CAD build for the part. Positions are in the model's coordinates, mm. A direction names the side the tool comes from. Coordinates: 2 decimals unless noted, no trailing zeros. Order: outer loops, then holes, each group sorted by start corner. A loop starts at its lowest first (then second) coordinate and runs counter-clockwise, first axis right, second up. Notation, with made-up numbers: M 49.5,-37.5 L 59.5,-37.5 A10 cw 59.5,-29.5 Z; hole C 9.5,35 d2. An arc over 180 degrees is marked long. One line per item, written item: value.
Autodesk Inventor part; units mm, degrees
ref_plane "YZ Plane" through (0, 0, 0) normal (1, 0, 0) x (0, 1, 0)
ref_plane "XZ Plane" through (0, 0, 0) normal (0, 1, 0) x (-1, 0, 0)
ref_plane "XY Plane" through (0, 0, 0) normal (0, 0, 1) x (1, 0, 0)
sketch "Sketch2" plane through (0, 0, 0) normal (0, 0, 1) x (1, 0, 0)
  line L0 (-7, 4.75) -> (12.8, 4.75)
  line L1 (12.8, 4.75) -> (12.8, -4.75)
  line L2 (12.8, -4.75) -> (-7, -4.75)
  line L3 (-7, -4.75) -> (-7, 4.75)
  line L4 (-3.9, 4.75) -> (0.1, 4.75)
  line L5 (0.1, 4.75) -> (0.1, 5.15)
  line L6 (0.1, 5.15) -> (-3.9, 5.15)
  line L7 (-3.9, 5.15) -> (-3.9, 4.75)
  line L8 (5.6, 4.75) -> (9.6, 4.75)
  line L9 (9.6, 4.75) -> (9.6, 5.15)
  line L10 (9.6, 5.15) -> (5.6, 5.15)
  line L11 (5.6, 5.15) -> (5.6, 4.75)
  line L12 (-7, -4.75) -> (3, -4.75)
  line L13 (3, -4.75) -> (3, -5.45)
  line L14 (3, -5.45) -> (-7, -5.45)
  line L15 (-7, -5.45) -> (-7, -4.75)
  circle A0 centre (-1.9, 2.25) radius 1.15
  circle A1 centre (7.6, 2.25) radius 1.15
  point P0 (0, 0)
  dimension "d2" = 19.8
  dimension "d3" = 9.5
  dimension "d4" = 7
  dimension "d5" = 4.75
  dimension "d6" = 0.4
  dimension "d8" = 0.4
  dimension "d10" = 4
  dimension "d11" = 4
  dimension "d13" = 10
  dimension "d14" = 5.1
  dimension "d15" = 9.5
  dimension "d16" = 2
  dimension "d17" = 2
  dimension "d18" = 3.2
  dimension "d21" = 2.3
  dimension "d22" = 2.3
  dimension "d80" = 7.2
  dimension "d81" = 2.5
  dimension "d82" = 2.5
  dimension "d83" = 10.2
extrude "Extrusion1" add sketch "Sketch2" along normal mid plane 6
chamfer "Chamfer1" distance 0.4 angle 45 4 edges at (-3.9, 5.15, 0) (0.1, 5.15, 0) (5.6, 5.15, 0) (9.6, 5.15, 0)
chamfer "Chamfer3" distance 0.7 angle 45 1 edges at (3, -5.45, 0)
sketch "Sketch3" plane through (0, 0, 3) normal (0, 0, 1) x (1, 0, 0)
  line L0 (9.2, 5.15) -> (9.6, 4.75)
  line L1 (9.6, 5.15) -> (5.6, 5.15)
  line L2 (5.6, 4.75) -> (6, 5.15)
  line L3 (-0.3, 5.15) -> (0.1, 4.75)
  line L4 (0.1, 5.15) -> (-3.9, 5.15)
  line L5 (-3.9, 4.75) -> (-3.5, 5.15)
  circle A0 centre (7.6, 2.25) radius 1.15
  circle A1 centre (-1.9, 2.25) radius 1.15
  circle A2 centre (-1.9, 2.25) radius 2
  circle A3 centre (7.6, 2.25) radius 2
  line L6 (-3.9, 2.25) -> (-3.9, 4.75)
  line L7 (0.1, 2.25) -> (0.1, 4.75)
  line L8 (5.6, 2.25) -> (5.6, 4.75)
  line L9 (9.6, 2.25) -> (9.6, 4.75)
  point P0 (0, 0)
  dimension "d28" = 4
  dimension "d29" = 4
  dimension "d30" = 4
extrude "Extrusion2" add sketch "Sketch3" along normal blind 0.2
mirror "Mirror1" about plane through (0, 0, 0) normal (0, 0, 1) of "Extrusion2"
sketch "Sketch4" plane through (-7, -5.45, -3) normal (0, -1, 0) x (1, 0, 0)
  line L0 (6, 5) -> (8, 5)
  line L1 (8, 5) -> (8, 1)
  line L2 (8, 1) -> (6, 1)
  line L3 (6, 1) -> (6, 5)
  point P0 (7, 3)
  dimension "d33" = 2
  dimension "d34" = 4
  dimension "d35" = 1
  dimension "d36" = 2
extrude "Extrusion3" cut sketch "Sketch4" against normal blind 4
sketch "Sketch5" plane through (-7, 4.75, 3) normal (0, 1, 0) x (1, 0, 0)
  line L0 (7.1, 6) -> (12.6, 6)
  line L1 (12.6, 0) -> (7.1, 0)
  line L2 (19.6, 0) -> (16.4, 0)
  line L3 (16.4, 6) -> (19.6, 6)
  line L4 (1.3, 4.7) -> (1.8, 4.7)
  line L5 (1.8, 4.7) -> (1.8, 1.3)
  line L6 (1.8, 1.3) -> (1.3, 1.3)
  line L7 (1.3, 1.3) -> (1.3, 4.7)
  line L8 (10.1, 4.7) -> (10.6, 4.7)
  line L9 (10.6, 4.7) -> (10.6, 1.3)
  line L10 (10.6, 1.3) -> (10.1, 1.3)
  line L11 (10.1, 1.3) -> (10.1, 4.7)
  line L12 (-0.2, 3) -> (19.6, 3) construction
  line L13 (17.4, 4.7) -> (17.9, 4.7)
  line L14 (17.9, 4.7) -> (17.9, 1.3)
  line L15 (17.9, 1.3) -> (17.4, 1.3)
  line L16 (17.4, 1.3) -> (17.4, 4.7)
  line L17 (0, 0) -> (0, 6)
  line L18 (0, 6) -> (3.1, 6)
  line L19 (0, 0) -> (0, 6)
  line L20 (19.8, 0) -> (16.6, 0)
  line L21 (19.8, 6) -> (19.8, 0)
  line L22 (0, 6) -> (3.1, 6)
  line L23 (3.1, 0) -> (3.1, 6)
  line L24 (3.1, 0) -> (0, 0)
  line L25 (12.6, 0) -> (12.6, 6)
  line L26 (7.1, 6) -> (12.6, 6)
  line L27 (7.1, 6) -> (7.1, 0)
  line L28 (12.6, 0) -> (7.1, 0)
  line L29 (16.4, 6) -> (16.4, 0)
  line L30 (3.1, 0) -> (3.1, 6)
  line L31 (3.1, 0) -> (0, 0)
  line L32 (12.6, 0) -> (12.6, 6)
  line L33 (7.1, 6) -> (7.1, 0)
  line L34 (16.6, 6) -> (16.6, 0)
  line L35 (16.6, 6) -> (19.8, 6)
  line L36 (3.1, 0) -> (0.4, 0)
  line L37 (1.55, 4.7) -> (1.55, 1.3) construction
  line L38 (10.35, 4.7) -> (10.35, 1.3) construction
  line L39 (17.65, 4.7) -> (17.65, 1.3) construction
  point P0 (7, 3)
  dimension "d39" = 3.4
  dimension "d40" = 3.4
  dimension "d41" = 0.5
  dimension "d42" = 0.5
  dimension "d43" = 1.7
  dimension "d44" = 1.7
  dimension "d46" = 9.3
  dimension "d47" = 3.4
  dimension "d48" = 0.5
  dimension "d49" = 1.7
  dimension "d50" = 16.6
  dimension "d87" = 8.8
  dimension "d88" = 7.3
  dimension "d89" = 3.1
  dimension "d90" = 1.55
  dimension "d91" = 6
  dimension "d92" = 3
extrude "Extrusion4" add sketch "Sketch5" along normal blind 4 contours L4 L5 L6 L7 | L8 L9 L10 L11 | L13 L14 L15 L16
chamfer "Chamfer2" distance 0.5 angle 45 6 edges at (-5.45, 8.75, 1.7) (-5.45, 8.75, -1.7) (3.35, 8.75, -1.7) (3.35, 8.75, 1.7) (10.65, 8.75, -1.7) (10.65, 8.75, 1.7)
sketch "Sketch6" plane through (-5.7, 4.75, -1.7) normal (-1, 0, 0) x (0, 0, 1)
  line L0 (0, 0) -> (0, 3.5)
  line L1 (3.4, 0) -> (3.4, 3.5)
  line L2 (0.5, 4) -> (2.9, 4)
  point P0 (1.7, -4.75)
  point P1 (1.7, 2.5)
  dimension "d56" = 3.4
  dimension "d57" = 1.7
  dimension "d58" = 1.5
hole "Hole1" at (-5.7, 7.25, 0) direction (1, 0, 0) diameter 1.6 end through all
sketch "Sketch7" plane through (0, 0, 3) normal (0, 0, 1) x (1, 0, 0)
  line L0 (-7, 4.75) -> (-7, -5.45)
  line L1 (-7, -5.45) -> (3, -5.45)
  line L2 (-4, -5.45) -> (-4, -2.45) construction
  line L3 (-5.5, -5.45) -> (-5.5, -2.45)
  line L4 (-2.5, -2.45) -> (-2.5, -5.45)
  arc A0 (-5.5, -5.45) -> (-2.5, -5.45) centre (-4, -5.45) ccw
  arc A1 (-2.5, -2.45) -> (-5.5, -2.45) centre (-4, -2.45) ccw
  point P0 (2.6, -5.45)
  point P1 (0, 0)
  point P2 (-4, -3.95)
  dimension "d66" = 3
  dimension "d68" = 3
  dimension "d69" = 3
extrude "Extrusion5" cut sketch "Sketch7" against normal blind 0.5
sketch "Sketch8" plane through (0, 0, 2.5) normal (0, 0, 1) x (1, 0, 0)
  arc A0 (-2.5, -2.45) -> (-5.5, -2.45) centre (-4, -2.45) ccw
  circle A1 centre (-4, -2.45) radius 0.4
  point P0 (0, 0)
  dimension "d72" = 0.8
extrude "Extrusion6" add sketch "Sketch8" along normal up to surface (0.5 mm away)
mirror "Mirror2" about plane through (0, 0, 0) normal (0, 0, 1) of "Extrusion5", "Extrusion6"
sketch "Sketch9" plane through (0, 0, -3) normal (0, 0, -1) x (-1, 0, 0)
  arc A0 (5.5, -2.45) -> (2.5, -2.45) centre (4, -2.45) ccw
  line L0 (5.5, -2.45) -> (5.5, -5.45)
  line L1 (5.5, -5.45) -> (7, -5.45)
  line L2 (6.0521, -5.45) -> (5.4772, -2.1895)
  line L3 (6.0521, -5.45) -> (5.5, -5.45)
  point P0 (0, 0)
  dimension "d75" = 10
extrude "Extrusion7" cut sketch "Sketch9" against normal up to surface (0.5 mm away)
mirror "Mirror3" about plane through (0, 0, 0) normal (0, 0, 1) of "Extrusion7"
fillet "Fillet1" radius 0.5 2 edges at (12.8, -4.75, 0) (-7, -5.45, 0)
equation "\"d8\" = d6"
equation "\"d11\" = d10"
equation "\"d22\" = d21"
equation "\"d29\" = d28"
equation "\"d30\" = d29"
equation "\"d40\" = d39"
equation "\"d42\" = d41"
equation "\"d43\" = 0.5 * d39"
equation "\"d44\" = 0.5 * d40"
equation "\"d47\" = d39"
equation "\"d48\" = d41"
equation "\"d49\" = 0.5 * d47"
equation "\"d90\" = 0.5 * d89"
equation "\"d92\" = 0.5 * d91"
properties part number "KW-5A-125250V_body#" material "PC_ABS Plastic"
Q1. Drill centre lines: line 1 along Y through (x, z) = (10.5, 0); line 2 along Z through (x, y) = (3.45, 7.25); line 3 along Z through (x, y) = (0, -2.5). Where is each one in solid material? Low to high.
Recorded:
line 1: y = -4.75 to 6.45, 8.05 to 8.75
line 2: z = -1.7 to -0.8, 0.8 to 1.7
line 3: z = -3 to -2, 2 to 3
Q2. Slice it at C-C (y = 1.5). List the corners of the cut face in (x, z).
Recorded:
outline: M -7,-3 L -3.75,-3 L -3.75,-3.2 L -2.77,-3.2 L -2.77,3.2 L -3.75,3.2 L -3.75,3 L -7,3 Z; M -1.03,-3.2 L -0.05,-3.2 L -0.05,-3 L 5.75,-3 L 5.75,-3.2 L 6.73,-3.2 L 6.73,3.2 L 5.75,3.2 L 5.75,3 L -0.05,3 L -0.05,3.2 L -1.03,3.2 Z; M 8.47,-3.2 L 9.45,-3.2 L 9.45,-3 L 12.8,-3 L 12.8,3 L 9.45,3 L 9.45,3.2 L 8.47,3.2 Z
Q3. Slice it at A-A (x = 8). List the corners of the cut face in (y, z).
Recorded:
outline: M -4.75,-3 L 0.29,-3 L 0.29,-3.2 L 1.17,-3.2 L 1.17,3.2 L 0.29,3.2 L 0.29,3 L -4.75,3 Z; M 3.33,-3.2 L 5.15,-3.2 L 5.15,3.2 L 3.33,3.2 Z
Q4. Pin check, flat tips, straight feed: pin 1 Ø1.4 at (y, z) = (7.25, 0) entering from +X; pin 2 Ø1.6 at (x, y) = (0, -4) entering from +Z; pin 3 Ø3 at (x, y) = (-5, -3) entering from -Z; pin 4 Ø4 at (x, y) = (2, 4) entering from +Z. Stop position of each tip, or through.
Recorded:
pin 1: passes through
pin 2: stops at z = 3
pin 3: stops at z = -3
pin 4: stops at z = 3.2
Q5. Which spindle directions (+Z, -Z, +X, -X, +Y, -Y) get a long thin tool onto all of the face, cutting with end or side? Do faces 1 (the face through (0, -3, 2)), 2 (the face through (-5.2, 6, 0)), 3 (the face through (3, 0, 3)). Say none if no direction does.
Recorded:
face 1: -Y
face 2: +Z, -Z, +Y
face 3: +Z, -Y
Q6. Slice it at B-B (z = 2.25). Give the number of separate pieces and of enclosed holes in the cut face, plus the area to 3 significant figures.
Recorded:
separate pieces: 1
enclosed holes: 2
area: 189 mm^2
Q7. Mould opens along Y. For faces 4 (the face through (-2, -5.45, 0)), 5 (the face through (-5.446, 6.457, -0.104)), 6 (the face through (8, 5.15, 0)), 7 (the face through (-2, 4, -3.2)) say: released by +Y, released by -Y, zero draft, split by the parting line, or undercut.
Recorded:
face 4: released by -Y
face 5: undercut
face 6: released by +Y
face 7: zero draft
